Part model, mm, in its own coordinate system. A direction names the side the tool comes from. Round coordinates to 2 decimals unless told otherwise and drop trailing zeros. Loops run counter-clockwise (first coordinate to the right, second up) from the corner with the lowest first, then second, coordinate; pieces in that order, holes last.
(1) Cut at B-B on x = 28. List the corners of the cut face in (y, z), then the cut area to 3 significant figures.
(2) Mould opens along X. For faces 3 (the face through (0, 0, 0)), 4 (the face through (-33.57, 8.5, 0.51)), 5 (the face through (-4, -5, 3.7)), 6 (the face through (-29.4, 0.06, 8.3)) say: +X half, -X half, draft (parallel to the pull), parting line (faces both ways), or undercut.
(3) Cut at D-D on z = 13.25. List the corners of the cut face in (x, y).
(4) Tool access for faces 1 (the face through (0, 10, 3)), 2 (the face through (1.9, -6.2, 5.8)): list every direction of +Z, -Z, +X, -X, +Y, -Y with a clear straight run to the whole face (end or side of a thin tool).
(5) Probe probe 1 along Y at (x, z) = (28, 0.75); probe 2 along Z at (x, y) = (-11, -3.25); probe 3 along X at (y, z) = (6.25, 8.25). List the from-to ranges inside material, lowest first.
(6) Flat gauge pins, fed straight in: pin 1 (4.5 mm diameter, centred on x = 3.5, y = -5, fed in from +Z); pin 2 (4.5 mm diameter, centred on x = -4, y = 4.5, fed in from +Z); pin 3 (1 mm diameter, centred on y = 0.5, z = 12.5, fed in from +X). Where does each tip first touch, or does it go through?
(7) Cut at A-A on z = 7. List the corners of the cut face in (x, y).
(8) Cut at C-C on x = 3.5. List the corners of the cut face in (y, z).
from build123d import *
from build123d import SkipClean  # not in build123d's __all__

# Parameters (mm, degrees)
F0_W      = 70
F0_H      = 20
F1_DEPTH  = 1
F3_D      = 3
F4_R      = 5
F7_DEPTH  = 0.5
F9_DEPTH  = 69.001
F10_W     = 16
F10_H     = 9.25
F10_H_2   = 1.5
F11_DEPTH = 6.9
F12_R     = 1.95
F13_DEPTH = 4
F14_R     = 2
F15_DEPTH = 4.2
F16_R     = 1.5
F17_DEPTH = 1
F18_R     = 1.4
F19_DEPTH = 14.8


with BuildPart() as f1:
    # F0 (on Top) → F1 (new body)
    with BuildSketch(Plane.XY):
        Rectangle(F0_W, F0_H)
    extrude(amount=F1_DEPTH)

    # F3 (through all)
    with Locations(Plane.XY.offset(1)):
        with Locations((-28, 0), (28, 0)):
            Hole(F3_D / 2)

    # F4
    f4_edges = [f1.edges().sort_by_distance(p)[0] for p in [
        (-35, 10, 0.5),
        (-35, -10, 0.5),
        (35, 10, 0.5),
        (35, -10, 0.5),
    ]]
    fillet(f4_edges, radius=F4_R)

    # F5 (on face) + F6 (on face) → F7 (join)
    with BuildSketch(Plane.XY.offset(1)):
        with BuildLine():
            Line((-29.2990381057, 0.75), (-34, 0.75))
            Line((-34, 0.75), (-34, -0.75))
            Line((-34, -0.75), (-29.2990381057, -0.75))
            ThreePointArc((-29.2990381057, -0.75), (-29.5, 0), (-29.2990381057, 0.75))
        make_face()
        with BuildLine():
            Line((-22, 0.75), (-26.7009618943, 0.75))
            ThreePointArc((-26.7009618943, 0.75), (-26.5511112606, 0.3882285677), (-26.5, 0))
            ThreePointArc((-26.5, 0), (-26.5511112606, -0.3882285677), (-26.7009618943, -0.75))
            Line((-26.7009618943, -0.75), (-22, -0.75))
            Line((-22, -0.75), (-22, 0.75))
        make_face()
    with BuildSketch(Plane.XY.offset(1)):
        with BuildLine():
            Line((26.7009618943, 0.75), (22, 0.75))
            Line((22, 0.75), (22, -0.75))
            Line((22, -0.75), (26.7009618943, -0.75))
            ThreePointArc((26.7009618943, -0.75), (26.5, 0), (26.7009618943, 0.75))
        make_face()
        with BuildLine():
            Line((34, 0.75), (29.2990381057, 0.75))
            ThreePointArc((29.2990381057, 0.75), (29.4488887394, 0.3882285677), (29.5, 0))
            ThreePointArc((29.5, 0), (29.4488887394, -0.3882285677), (29.2990381057, -0.75))
            Line((29.2990381057, -0.75), (34, -0.75))
            Line((34, -0.75), (34, 0.75))
        make_face()
    with SkipClean():  # cleaning this boolean's faces spoils the solid; the shape is the same uncleaned
        extrude(amount=F7_DEPTH)

    # F8 (on face) → F9 (cut, through all)
    with BuildSketch(Plane(origin=(-34, 0, 0), x_dir=(0, -1, 0), z_dir=(-1, 0, 0))):
        Polygon((-0.75, 1.5), (-0.75, 1), (0, 1.5), align=None)
        Polygon((0.75, 1.5), (0, 1.5), (0.75, 1), align=None)
    with SkipClean():  # cleaning this boolean's faces spoils the solid; the shape is the same uncleaned
        extrude(amount=-F9_DEPTH, mode=Mode.SUBTRACT)

    # F10 (on face) → F11 (join)
    with BuildSketch(Plane.XY.offset(1)):
        with Locations((0, -5.375)):
            Rectangle(F10_W, F10_H)
        Rectangle(F10_W, F10_H_2)
        with Locations((0, 5.375)):
            Rectangle(F10_W, F10_H)
    with SkipClean():  # cleaning this boolean's faces spoils the solid; the shape is the same uncleaned
        extrude(amount=F11_DEPTH)

    # F12 (on face) → F13 (join)
    with BuildSketch(Plane.XY.offset(7.9)):
        with Locations((-3.5, 5)):
            Circle(F12_R)
        with Locations((3.5, 5)):
            Circle(F12_R)
    with SkipClean():  # cleaning this boolean's faces spoils the solid; the shape is the same uncleaned
        extrude(amount=F13_DEPTH)

    # F14 (on face) → F15 (cut)
    with BuildSketch(Plane.XY.offset(7.9)):
        with Locations((-3.5, -5)):
            Circle(F14_R)
        with Locations((3.5, -5)):
            Circle(F14_R)
    with SkipClean():  # cleaning this boolean's faces spoils the solid; the shape is the same uncleaned
        extrude(amount=-F15_DEPTH, mode=Mode.SUBTRACT)

    # F16 (on face) → F17 (join)
    with BuildSketch(Plane.XY.offset(1)):
        with Locations((-28, 0)):
            Circle(F16_R)
    with SkipClean():  # cleaning this boolean's faces spoils the solid; the shape is the same uncleaned
        extrude(amount=-F17_DEPTH)

    # F18 (on face) → F19 (join)
    with BuildSketch(Plane.XY.offset(1)):
        with Locations((-28, 0)):
            Circle(F18_R)
    with SkipClean():  # cleaning this boolean's faces spoils the solid; the shape is the same uncleaned
        extrude(amount=F19_DEPTH)


solid = f1.part
Final values:
1. outline: (-10, 0) - (-1.5, 0) - (-1.5, 1) - (-10, 1) - close; (1.5, 0) - (10, 0) - (10, 1) - (1.5, 1) - close
1. area: 17.0 mm2
2. face 3: draft
2. face 4: -X half
2. face 5: undercut
2. face 6: undercut
3. outline: circle Ø2.8 at (-28, 0)
4. face 1: +Z, -Z, +X, -X, +Y
4. face 2: +Z
5. probe 1: y = -10 to -1.5, 1.5 to 10
5. probe 2: z = 0 to 1
5. probe 3: x = -5 to -2, 2 to 5
6. pin 1: stops at z = 7.9
6. pin 2: stops at z = 11.9
6. pin 3: stops at x = -26.6
7. outline: circle Ø2.8 at (-28, 0); (-8, -10) - (8, -10) - (8, 10) - (-8, 10) - close; hole circle Ø4 at (-3.5, -5); hole circle Ø4 at (3.5, -5)
8. outline: (-10, 0) - (10, 0) - (10, 7.9) - (6.95, 7.9) - (6.95, 11.9) - (3.05, 11.9) - (3.05, 7.9) - (-3, 7.9) - (-3, 3.7) - (-7, 3.7) - (-7, 7.9) - (-10, 7.9) - close
